Autodesk Inventor part; units mm, degrees
ref_plane "YZ Plane" through (0, 0, 0) normal (1, 0, 0) x (0, 1, 0)
ref_plane "XZ Plane" through (0, 0, 0) normal (0, 1, 0) x (-1, 0, 0)
ref_plane "XY Plane" through (0, 0, 0) normal (0, 0, 1) x (1, 0, 0)
sketch "Sketch1" plane through (0, 0, 0) normal (1, 0, 0) x (0, 1, 0)
  line L0 (0, 0) -> (482.6, 0)
  line L1 (482.6, 0) -> (482.6, -19.05)
  line L2 (482.6, -19.05) -> (0, -19.05)
  line L3 (0, -19.05) -> (0, 0)
  circle A0 centre (469.9, -9.525) radius 6.35
  circle A1 centre (12.7, -9.525) radius 6.35
  dimension "d0" = 482.6
  dimension "d1" = 19.05
  dimension "d2" = 12.7
  dimension "d3" = 12.7
  dimension "d4" = 12.7
  dimension "d5" = 12.7
extrude "Extrusion1" add sketch "Sketch1" along normal blind 50.8
equation "\"d5\" = d4"
properties part number "ArmProto"
The listing builds one solid part. Answer for the finished solid, in the listing's coordinates (mm). Give positions to 0.01 mm unless a question says otherwise; leave off trailing zeros. Write each loop counter-clockwise with the first axis right and the second up, starting at its lowest first coordinate (ties: lowest second). Pieces come first, ordered by that corner, then holes.
Item 1: Section B-B, the plane x = 41.5 is taken. Write down the section's boundary in (y, z) (3 decimals).
Item 2: Find the intervals of material crossed by line 1 along Y through (x, z) = (39, -10.5); line 2 along Y through (x, z) = (26, -6.5); line 3 along Z through (x, y) = (33, 12.7) (3 decimals), in increasing order.
Item 3: Section A-A, the plane y = 12.7 is taken. Write down the section's boundary in (x, z) (3 decimals).
Item 4: A flat-ended cylindrical pin translates along its axis: P1, Ø10, axis at y = 469.9, z = -9.525, coming from the -X side. Find the tip coordinate at first contact, or state that the pin passes through.
Item 5: Determine the mould class of faces 1 (the flat face through (25, 0, -10)), 2 (the flat face through (25, 245, -19.05)), 3 (the cylindrical face through (25.044, 475.766, -7.093)) for opening direction Z: released by +Z, released by -Z, zero draft, split by the parting line, or undercut.
Completed:
1. outline: (0, -19.05) - (482.6, -19.05) - (482.6, 0) - (0, 0) - close; hole circle Ø12.7 at (12.7, -9.525); hole circle Ø12.7 at (469.9, -9.525)
2. line 1: y = 0 to 6.43, 18.97 to 463.63, 476.17 to 482.6
2. line 2: y = 0 to 7.12, 18.28 to 464.32, 475.48 to 482.6
2. line 3: z = -19.05 to -15.875, -3.175 to 0
3. outline: (0, -19.05) - (50.8, -19.05) - (50.8, -15.875) - (0, -15.875) - close; (0, -3.175) - (50.8, -3.175) - (50.8, 0) - (0, 0) - close
4. P1: passes through
5. face 1: zero draft
5. face 2: released by -Z
5. face 3: undercut
